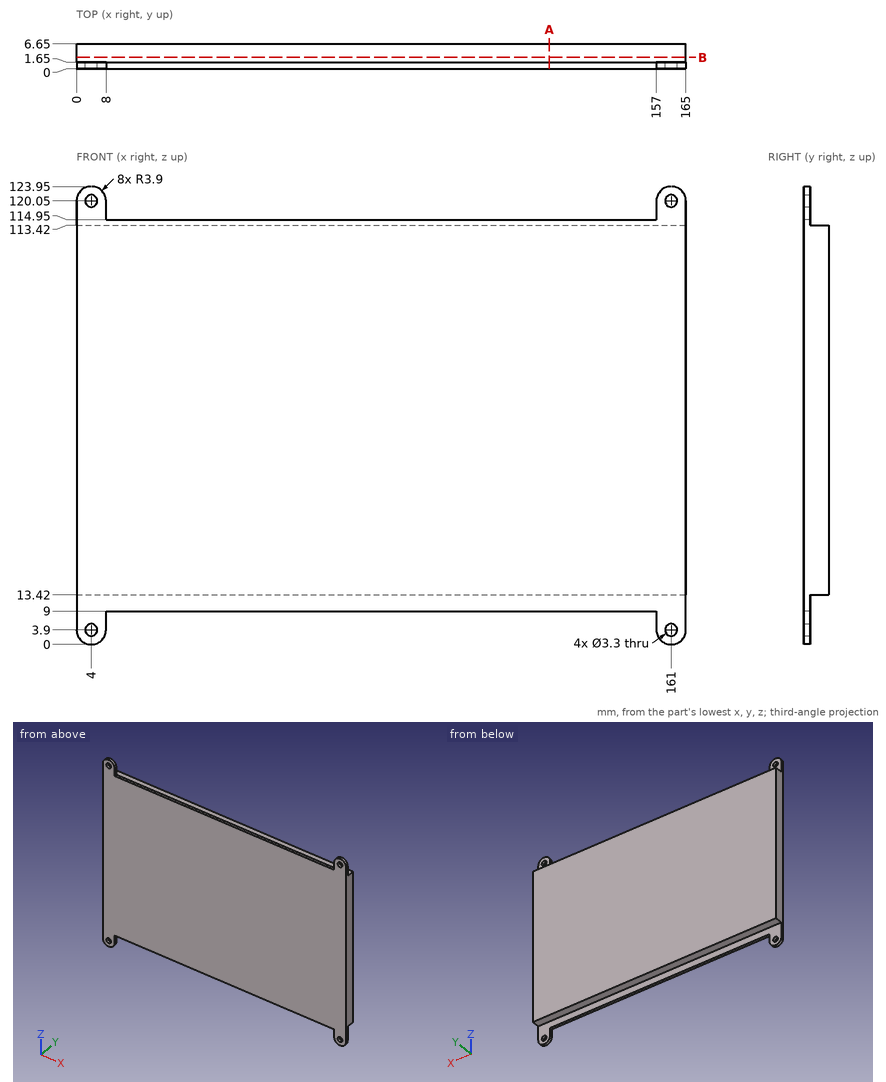
Print and shaded views of the part. All mm, measured from the part's lowest x, y and z. Round coordinates to 2 decimals unless told otherwise and drop trailing zeros. Write each loop counter-clockwise with the first axis right and the second up, starting at its lowest first coordinate (ties: lowest second). Pieces come first, ordered by that corner, then holes.
(1) Drop flat-ended pins along their axis: P1, Ø2.5, axis at x = 49, y = 3.5, coming from the -Z side; P2, Ø1.3, axis at y = 1, z = 117, coming from the -X side; P3, Ø10.5, axis at x = 42, z = 4.5, coming from the +Y side; P4, Ø0.8, axis at x = 85.5, y = 1, coming from the -Z side. Give the stop position or say it passes through.
(2) Slice it at B-B, the plane y = 3. Write the cut outline in (x, z), and give its area (3 significant figures).
(3) Probe line 1 along X through (y, z) = (0.75, 3.9); line 2 along Z through (x, y) = (161, 0.9); line 3 along Z through (x, y) = (109, 3.75). List the from-to ranges inside material, lowest first.
(4) Slice it at A-A, the plane x = 128. Write the cut outline in (y, z), and give its area (3 significant figures).
From the geometry:
1. P1: stops at z = 13.42
1. P2: stops at x = 0
1. P3: stops at y = 1.65
1. P4: stops at z = 9
2. outline: (0, 13.42) - (165, 13.42) - (165, 113.42) - (0, 113.42) - close
2. area: 16,500 mm2
3. line 1: x = 0 to 2.35, 5.65 to 8, 157 to 159.35, 162.65 to 165
3. line 2: z = 0 to 2.25, 5.55 to 118.4, 121.7 to 123.95
3. line 3: z = 13.42 to 113.42
4. outline: (0, 9) - (1.65, 9) - (1.65, 13.42) - (6.65, 13.42) - (6.65, 113.42) - (1.65, 113.42) - (1.65, 114.95) - (0, 114.95) - close
4. area: 675 mm2
